Could you check a few things on this model? Use its own coordinates, in mm. Give positions to 0.01 mm unless a question says otherwise; leave off trailing zeros. Order: outer loops, then holes, each group sorted by start corner. A loop starts at its lowest first (then second) coordinate and runs counter-clockwise, first axis right, second up. Notation, with made-up numbers: M 21.25,41.25 L 51.25,41.25 A28 cw 51.25,74.25 Z; hole C 69.25,-24 d7. An arc over 180 degrees is marked long. Use a Markdown table: item, result. Add a question column.
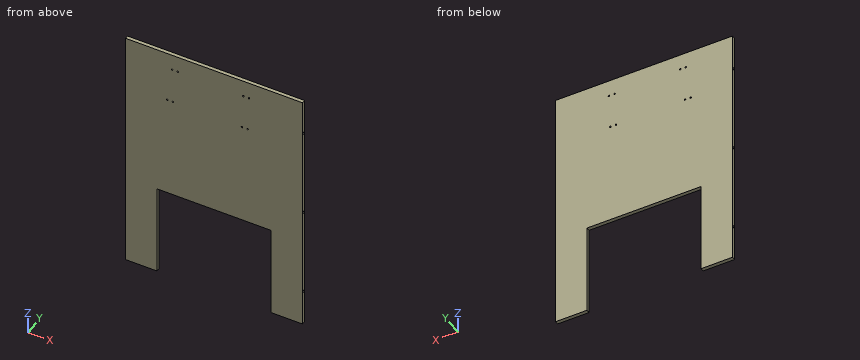
Autodesk Inventor part; units mm, degrees
ref_plane "YZ Plane" through (0, 0, 0) normal (1, 0, 0) x (0, 1, 0)
ref_plane "XZ Plane" through (0, 0, 0) normal (0, 1, 0) x (-1, 0, 0)
ref_plane "XY Plane" through (0, 0, 0) normal (0, 0, 1) x (1, 0, 0)
sketch "Sketch1" plane through (0, 0, 0) normal (0, 1, 0) x (-1, 0, 0)
  line L0 (0, 0) -> (314.96, 0)
  line L1 (314.96, 0) -> (314.96, -444.5)
  line L2 (314.96, -444.5) -> (0, -444.5)
  line L3 (0, -444.5) -> (0, 0)
  dimension "d0" = 314.96
  dimension "d1" = 444.5
extrude "Extrusion1" add sketch "Sketch1" along normal blind 6.35
sketch "Sketch2" plane through (0, 6.35, 0) normal (0, 1, 0) x (1, 0, 0)
  circle A0 centre (-95.1484, 30.099) radius 1.3589
  circle A1 centre (-105.156, 30.099) radius 1.3589
  line L0 (-314.96, 0) -> (0, 0)
  line L1 (0, 0) -> (0, 444.5)
  dimension "d4" = 2.7178
  dimension "d5" = 2.7178
  dimension "d7" = 95.1484
  dimension "d8" = 10.0076
  dimension "d9" = 30.099
  dimension "d37" = 30.099
extrude "Extrusion2" cut sketch "Sketch2" against normal blind 25.4
sketch "Sketch3" plane through (0, 6.35, 0) normal (0, 1, 0) x (1, 0, 0)
  circle A0 centre (-107.696, 93.1418) radius 1.3589
  circle A1 centre (-97.6884, 93.1418) radius 1.3589
  circle A2 centre (-95.1484, 30.099) radius 1.3589
  circle A3 centre (-105.156, 30.099) radius 1.3589
  line L0 (0, 0) -> (0, 444.5)
  dimension "d12" = 2.7178
  dimension "d13" = 2.7178
  dimension "d14" = 63.0428
  dimension "d15" = 63.0428
  dimension "d16" = 10.0076
  dimension "d17" = 97.6884
extrude "Extrusion3" cut sketch "Sketch3" against normal blind 25.4 contours A0 | A1
sketch "Sketch4" plane through (0, 6.35, 0) normal (0, 1, 0) x (1, 0, 0)
  circle A0 centre (-240.5634, 93.091) radius 1.3589
  circle A1 centre (-230.5562, 93.1789) radius 1.3589
  line L0 (-314.96, 444.5) -> (-314.96, 0)
  line L1 (-314.96, 0) -> (0, 0)
  dimension "d20" = 2.7178
  dimension "d21" = 2.7178
  dimension "d22" = 10.0076
  dimension "d23" = 74.3966
  dimension "d24" = 93.091
extrude "Extrusion4" cut sketch "Sketch4" against normal blind 25.4
sketch "Sketch5" plane through (0, 6.35, 0) normal (0, 1, 0) x (1, 0, 0)
  circle A0 centre (-232.029, 28.702) radius 1.3589
  circle A1 centre (-222.0214, 28.702) radius 1.3589
  line L0 (-314.96, 0) -> (0, 0)
  line L1 (-314.96, 444.5) -> (-314.96, 0)
  line L2 (0, 0) -> (0, 444.5)
  dimension "d27" = 2.7178
  dimension "d28" = 2.7178
  dimension "d31" = 28.702
  dimension "d32" = 10.0076
  dimension "d36" = 222.0214
  dimension "d38" = 28.702
extrude "Extrusion5" cut sketch "Sketch5" against normal blind 25.4
sketch "Sketch6" plane through (0, 0, 0) normal (1, 0, 0) x (0, 0, -1)
  line L0 (444.5, 0) -> (444.5, 6.35)
  line L1 (0, 6.35) -> (444.5, 6.35)
  line L2 (0, 0) -> (0, 6.35)
  point P0 (63.5, 3.175)
  point P1 (222.25, 3.175)
  point P2 (381, 3.175)
  dimension "d39" = 6.35
  dimension "d40" = 3.175
  dimension "d41" = 3.175
  dimension "d42" = 3.175
  dimension "d43" = 63.5
  dimension "d44" = 63.5
  dimension "d45" = 317.5
  dimension "d46" = 158.75
hole "Hole1" at (0, 3.175, -63.5) at (0, 3.175, -222.25) at (0, 3.175, -381) direction (-1, 0, 0) diameter 4.9784 depth 19.05 tip angle 118
ref_plane "Work Plane1" through (-157.48, 0, 0) normal (1, 0, 0) x (0, 0, -1)
mirror "Mirror1" about plane through (-157.48, 0, 0) normal (1, 0, 0) of "Hole1"
sketch "Sketch7" plane through (0, 6.35, 0) normal (0, 1, 0) x (1, 0, 0)
  line L0 (0, 444.5) -> (-314.96, 444.5)
  line L1 (-55.88, 444.5) -> (-259.08, 444.5)
  line L2 (-259.08, 444.5) -> (-259.08, 279.4)
  line L3 (-259.08, 279.4) -> (-55.88, 279.4)
  line L4 (-55.88, 279.4) -> (-55.88, 444.5)
  line L5 (-314.96, 444.5) -> (-314.96, 0)
  point P0 (0, 0)
  dimension "d54" = 203.2
  dimension "d55" = 165.1
  dimension "d56" = 55.88
extrude "Extrusion6" cut sketch "Sketch7" against normal through all
properties part number "main plate"
1) Suppose I cut it at B-B on x = -156. Please give me the cut outline in (y, z).
2) Suppose I cut it at C-C on y = 2. Count the separate pieces of the cut face and the enclosed holes in it, and give its area (3 significant figures).
3) For pin 1 (3 mm diameter, centred on y = 3.175, z = -63.5, fed in from +X); pin 2 (3.5 mm diameter, centred on x = -232.029, z = -28.702, fed in from -Y); pin 3 (1.9 mm diameter, centred on x = -171.5, y = 3.5, fed in from -Z), each with a flat end and sliding along its axis, tell me the tip position at first contact or that it passes through.
4) Please list where these lines run through material, in increasing order: line 1 (Z direction, x = -13, y = 2.5); line 2 (X direction, y = 5.25, z = -377); line 3 (Z direction, x = -119, y = 3). Write a range as from..to.
5) Suppose I cut it at A-A on z = -353.5. Please give me the cut outline in (x, y).
Values found:
| question | item | result |
|---|---|---|
| 1 | outline | M 0,-279.4 L 6.35,-279.4 L 6.35,0 L 0,0 Z |
| 2 | separate pieces | 1 |
| 2 | enclosed holes | 8 |
| 2 | area | 106,000 mm^2 |
| 3 | pin 1 | stops at x = -19.64 |
| 3 | pin 2 | stops at y = 0 |
| 3 | pin 3 | stops at z = -279.4 |
| 4 | line 1 | z = -444.5..-383.4, -378.6..-224.65, -219.85..-65.9, -61.1..0 |
| 4 | line 2 | x = -314.96..-259.08, -55.88..0 |
| 4 | line 3 | z = -279.4..0 |
| 5 | outline | M -314.96,0 L -259.08,0 L -259.08,6.35 L -314.96,6.35 Z; M -55.88,0 L 0,0 L 0,6.35 L -55.88,6.35 Z |
